Geometry: final body of the model. Coordinates: model frame, mm. Give positions to 0.01 mm unless a question says otherwise; leave off trailing zeros. Write each loop counter-clockwise with the first axis right and the second up, starting at its lowest first coordinate (ties: lowest second). Pieces come first, ordered by that corner, then holes.
```python
from build123d import *

# Parameters (mm, degrees)
F1_DEPTH = 19.05


# Not quite as in the source:
# - a feature names something its author has since deleted; it is built from what else it names


with BuildPart() as f1:
    # F0 (on Front) → F1 (new body)
    with BuildSketch(Plane.XZ):
        Polygon((-140.5185023113, -17.3581795608), (-115.1141719677, -17.3581795608), (-115.1141719677, -36.4081795608), (-102.4141719677, -36.4081795608), (-102.4141719677, -17.3581795608), (-64.3141719677, -17.3581795608), (-64.3141719677, -36.4081795608), (-51.6141719677, -36.4081795608), (-51.6141719677, -17.3581795608), (125.7340388179, -17.3581795608), (138.656257718, -4.8882621778), (138.656257718, 20.7418204392), (113.256257718, 20.7418204392), (113.256257718, 39.7918204392), (100.556257718, 39.7918204392), (100.556257718, 20.7418204392), (62.456257718, 20.7418204392), (62.456257718, 39.7918204392), (49.756257718, 39.7918204392), (49.756257718, 20.7418204392), (-128.043742282, 20.7418204392), (-140.5185023113, 8.2640567404), align=None)
    extrude(amount=F1_DEPTH)


solid = f1.part
```
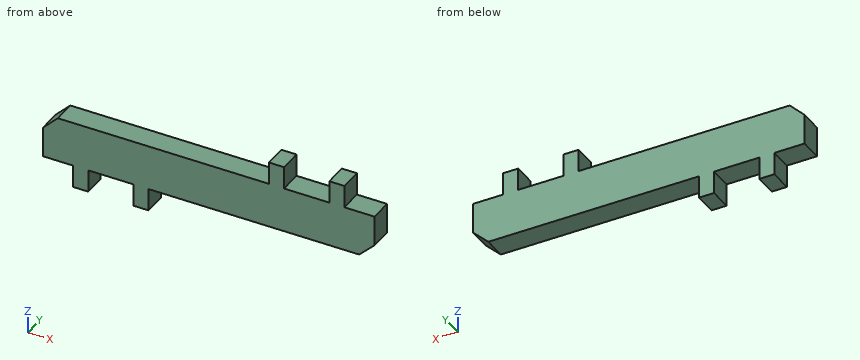
Item 1: Section D-D, the plane x = -105.5. Return the cut outline in (y, z).
Found:
outline: (-19.05, -36.41) - (0, -36.41) - (0, 20.74) - (-19.05, 20.74) - close
Item 2: Pin query (flat end, axial travel): pin 1 Ø5.5 at (x, y) = (121, -6) entering from +Z; pin 2 Ø5 at (x, z) = (24.5, -4.5) entering from +Y; pin 3 Ø9.5 at (y, z) = (-5.5, 26.5) entering from +X; pin 4 Ø5.5 at (x, y) = (-122, -8.5) entering from -Z. Return the tip coordinate at first contact, or that it passes through.
Found:
pin 1: stops at z = 20.74
pin 2: stops at y = 0
pin 3: stops at x = 113.26
pin 4: stops at z = -17.36
Item 3: Section C-C, the plane x = 10.5. Return the cut outline in (y, z).
Found:
outline: (-19.05, -17.36) - (0, -17.36) - (0, 20.74) - (-19.05, 20.74) - close
Item 4: Line query: L1, parallel to Z at x = 116, y = -17.25; L2, parallel to Z at x = 103, y = -2.5; L3, parallel to X at y = -14, z = 24. Output: solid intervals per line, ascending.
Found:
L1: z = -17.36 to 20.74
L2: z = -17.36 to 39.79
L3: x = 49.76 to 62.46, 100.56 to 113.26
Item 5: Section A-A, the plane z = 27.5. Return the cut outline in (x, y).
Found:
outline: (49.76, -19.05) - (62.46, -19.05) - (62.46, 0) - (49.76, 0) - close; (100.56, -19.05) - (113.26, -19.05) - (113.26, 0) - (100.56, 0) - close
Item 6: Section B-B, the plane y = -12.5. Return the cut outline in (x, z), plus the area to 3 significant figures.
Found:
outline: (-140.52, -17.36) - (-115.11, -17.36) - (-115.11, -36.41) - (-102.41, -36.41) - (-102.41, -17.36) - (-64.31, -17.36) - (-64.31, -36.41) - (-51.61, -36.41) - (-51.61, -17.36) - (125.73, -17.36) - (138.66, -4.89) - (138.66, 20.74) - (113.26, 20.74) - (113.26, 39.79) - (100.56, 39.79) - (100.56, 20.74) - (62.46, 20.74) - (62.46, 39.79) - (49.76, 39.79) - (49.76, 20.74) - (-128.04, 20.74) - (-140.52, 8.26) - close
area: 11,400 mm2
